Answer from the drawing. Dimensions are ordinates in mm from the lowest x, y and z of the part. A direction names the side the tool comes from. Give positions to 0.01 mm unless a question says otherwise; leave off trailing zeros. Order: outer loops, then holes, each group sorted by start corner. A loop starts at its lowest first (then second) coordinate and runs counter-clockwise, first axis right, second up. Notation, with made-up numbers: (-4, -8) - (47, -8) arc R19 cw to (47, 27) - close; hole circle Ø5 at (-19, 61.5). An arc over 180 degrees is marked (long way). Answer in a Markdown table with one row per item. Add a question column.
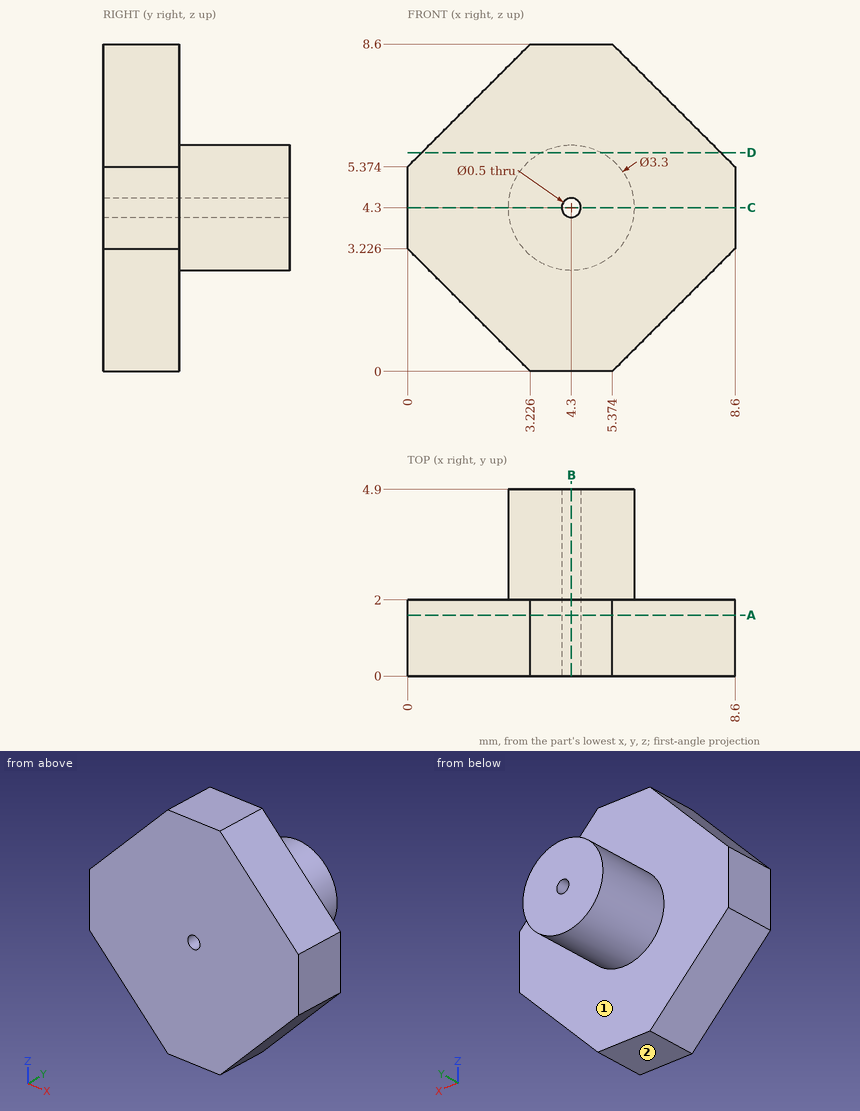
(1) Straight lines are drawn through the part: line 1 (X direction, y = 1.45, z = 4.3); line 2 (X direction, y = 3.3, z = 4.3); line 3 (Y direction, x = 5.75, z = 5.5). For each, find the intervals that lie inside material, in ascending order.
(2) For the marked faces 1 and 2, determine the directions among +Z, -Z, +X, -X, +Y, -Y from which every point of the face is accessible in a straight line to the end or side of a thin tool.
(3) Find section C-C, the plane z = 4.3. Write down the section's boundary in (x, y).
(4) Find section D-D, the plane z = 5.75. Write down the section's boundary in (x, y).
(5) Find section A-A, the plane y = 1.6. Write down the section's boundary in (x, z).
(6) Find section B-B, the plane x = 4.3. Write down the section's boundary in (y, z), plus the area to 3 significant figures.
(7) This flat-tipped pin is pushed along its axis until it touches: P1, Ø2, axis at x = 7.5, y = 1.5, coming from the +Z side. Where does it stop, or does it pass through?
Answer key:
| question | item | result |
|---|---|---|
| 1 | line 1 | 0 to 4.05, 4.55 to 8.6 |
| 1 | line 2 | 2.65 to 4.05, 4.55 to 5.95 |
| 1 | line 3 | 0 to 2 |
| 2 | face 1 | +Y |
| 2 | face 2 | -Z, +X, -X, +Y, -Y |
| 3 | outline | (0, 0) - (4.05, 0) - (4.05, 4.9) - (2.65, 4.9) - (2.65, 2) - (0, 2) - close; (4.55, 0) - (8.6, 0) - (8.6, 2) - (5.95, 2) - (5.95, 4.9) - (4.55, 4.9) - close |
| 4 | outline | (0.38, 0) - (8.22, 0) - (8.22, 2) - (5.09, 2) - (5.09, 4.9) - (3.51, 4.9) - (3.51, 2) - (0.38, 2) - close |
| 5 | outline | (0, 3.23) - (3.23, 0) - (5.37, 0) - (8.6, 3.23) - (8.6, 5.37) - (5.37, 8.6) - (3.23, 8.6) - (0, 5.37) - close; hole circle Ø0.5 at (4.3, 4.3) |
| 6 | outline | (0, 0) - (2, 0) - (2, 2.65) - (4.9, 2.65) - (4.9, 4.05) - (0, 4.05) - close; (0, 4.55) - (4.9, 4.55) - (4.9, 5.95) - (2, 5.95) - (2, 8.6) - (0, 8.6) - close |
| 6 | area | 24.3 mm² |
| 7 | P1 | z = 7.47 |
